CAD build for the part. Positions are in the model's coordinates, mm. A direction names the side the tool comes from. Round coordinates to 2 decimals unless told otherwise and drop trailing zeros. Write each loop counter-clockwise with the first axis right and the second up, starting at its lowest first coordinate (ties: lowest second). Pieces come first, ordered by that corner, then holes. Notation, with made-up numbers: (19, 13.25) -> (32, 13.25) arc R31 cw to (32, 48.25) -> close; hole circle Ø2 at (-30, -29.5). An arc over 180 degrees is marked (long way). Put each result on its own line as item: value. Start each with the question number.
1. Saw through at C-C on y = -10.25. List the corners of the cut face in (x, z) (3 decimals).
2. Drill centre lines: line 1 (X direction, y = -0.2, z = 8) (3 decimals); line 2 (X direction, y = 0.25, z = -8) (3 decimals); line 3 (X direction, y = -1.75, z = -7.25). Where is each one in solid material? Low to high. Write a range as from..to.
3. Saw through at A-A on y = -2.5. List the corners of the cut face in (x, z) (3 decimals).
4. Saw through at B-B on z = 0. List the corners of the cut face in (x, y) (3 decimals), and give its area (3 significant figures).
5. 3-axis set-ups, long thin cutter, end or side, ignore diameter. For faces 5 (the flat face through (11, -14, 0)), 6 (the cylindrical face through (0, -2.2, -4.5)), 7 (the cylindrical face through (-4.135, -7.162, 3.064)), 8 (the cylindrical face through (0, -2.2, -9.5)), 9 (the flat face through (0, -3.5, -7)): which of +Z, -Z, +X, -X, +Y, -Y reach the whole face in a straight line?
6. Flat gauge pins, fed straight in: P1, Ø4, axis at x = 15, y = -4, coming from the +Z side; P2, Ø3, axis at x = 0, z = -7.5, coming from the -Y side; P3, Ø5, axis at x = -19.525, z = -8, coming from the -Y side. Where does each tip first touch, or does it go through?
7. Saw through at D-D on z = 8.75. List the corners of the cut face in (x, y) (3 decimals).
8. Pull direction X, two halves, no side cores. Call faces 1 (the flat face through (0, -1, 0)), 2 (the flat face through (21.525, 0, 0)), 3 (the flat face through (-1.777, -2, -7)), 4 (the flat face through (0, 1, 0)): pulls with the +X half, pulls with the -X half, needs draft (parallel to the pull), parting line crosses it, or undercut.
from build123d import *

# Parameters (mm, degrees)
SCHIZZO1_W                   = 43.05
SCHIZZO1_H                   = 20
ESTRUSIONE_ESTRUSIONE1_DEPTH = 2
ESTRUSIONE_ESTRUSIONE2_DEPTH = 2.5
SCHIZZO3_W                   = 8
SCHIZZO3_H                   = 13
SCHIZZO4_W                   = 8
SCHIZZO4_H                   = 13
FORO_3_0_3_1_D               = 3
FORO_3_0_3_1_DEPTH           = 15
RACCORDO1_R                  = 0.5


with BuildPart() as part:
    # Schizzo1 → Estrusione-Estrusione1 (new body)
    with BuildSketch(Plane.XZ.offset(1)):
        Rectangle(SCHIZZO1_W, SCHIZZO1_H)
    extrude(amount=-ESTRUSIONE_ESTRUSIONE1_DEPTH)

    # Schizzo2 → Estrusione-Estrusione2 (add)
    with BuildSketch(Plane.XZ.offset(1)):
        with BuildLine():
            Line((-1.776510899, -8.758979541), (-1.776510899, -5.241020459))
            ThreePointArc((-1.776510899, -5.241020459), (0.01258154, -4.500031659), (1.794125223, -5.258990326))
            Line((1.794125223, -5.258990326), (1.794125223, -8.741009674))
            ThreePointArc((1.794125223, -8.741009674), (0.01258154, -9.499968341), (-1.776510899, -8.758979541))
        make_face()
    extrude(amount=ESTRUSIONE_ESTRUSIONE2_DEPTH)

    # Schizzo3 → Rivoluzione1 (revolve)
    with BuildSketch(Plane(origin=(0, 0, 0), x_dir=(-1, 0, 0), z_dir=(0, 0, -1))):
        with Locations((7.525, -7.5)):
            Rectangle(SCHIZZO3_W, SCHIZZO3_H)
    revolve(axis=Axis((-11.525, -14, 0), (0, 1, 0)))

    # Schizzo4 → Rivoluzione2 (revolve)
    with BuildSketch(Plane(origin=(0, 0, 0), x_dir=(-1, 0, 0), z_dir=(0, 0, -1))):
        with Locations((-15.525, -7.5)):
            Rectangle(SCHIZZO4_W, SCHIZZO4_H)
    revolve(axis=Axis((11.525, -14, 0), (0, 1, 0)))

    # Foro Ø3.0 (3)-1
    with Locations(Plane(origin=(0, 1, 0), x_dir=(1, 0, 0), z_dir=(0, 1, 0))):
        with Locations((-19.525, 8), (19.525, -8)):
            Hole(FORO_3_0_3_1_D / 2, depth=FORO_3_0_3_1_DEPTH)

    # Raccordo1
    raccordo1_edges = [part.edges().sort_by_distance(p)[0] for p in [
        (-19.525, -14, 0),
        (3.525, -14, 0),
    ]]
    fillet(raccordo1_edges, radius=RACCORDO1_R)


solid = part.part
Return value:
1. outline: circle Ø16 at (-11.525, 0); circle Ø16 at (11.525, 0)
2. line 1: x = -21.525..18.025, 21.025..21.525
2. line 2: x = -21.525..-21.025, -18.025..21.525
2. line 3: x = -14.91..-8.14, -1.78..1.79, 8.14..14.91
3. outline: circle Ø16 at (-11.525, 0); (-1.777, -8.759) arc R2.5 ccw to (1.794, -8.741) -> (1.794, -5.259) arc R2.5 ccw to (-1.777, -5.241) -> close; circle Ø16 at (11.525, 0)
4. outline: (-21.525, -1) -> (-19.525, -1) -> (-19.525, -13.5) arc R0.5 ccw to (-19.025, -14) -> (-4.025, -14) arc R0.5 ccw to (-3.525, -13.5) -> (-3.525, -1) -> (3.525, -1) -> (3.525, -13.5) arc R0.5 ccw to (4.025, -14) -> (19.025, -14) arc R0.5 ccw to (19.525, -13.5) -> (19.525, -1) -> (21.525, -1) -> (21.525, 1) -> (-21.525, 1) -> close
4. area: 502 mm^2
5. face 5: +Z, -Z, +X, -X, -Y
5. face 6: +Z, -Y
5. face 7: -Y
5. face 8: -Z, -Y
5. face 9: +Z, -Z, -Y
6. P1: stops at z = 7.86
6. P2: stops at y = -3.5
6. P3: stops at y = -1
7. outline: (-21.525, -1) -> (18.226, -1) -> (18.226, 1) -> (-21.525, 1) -> close; (20.824, -1) -> (21.525, -1) -> (21.525, 1) -> (20.824, 1) -> close
8. face 1: undercut
8. face 2: pulls with the +X half
8. face 3: undercut
8. face 4: needs draft
